Part print with two shaded views. Sizes in mm from the minimum x, y, z corner. Coordinates: 2 decimals unless noted, no trailing zeros. Loops run counter-clockwise (first coordinate to the right, second up) from the corner with the lowest first, then second, coordinate; pieces in that order, holes last. Notation, with made-up numbers: (24, 78.25) -> (57, 78.25) arc R7 cw to (57, 88.25) -> close; hole circle Ø1 at (-34, 76.25). An arc over 180 degrees is marked (long way). Use one line per item in the form item = value.
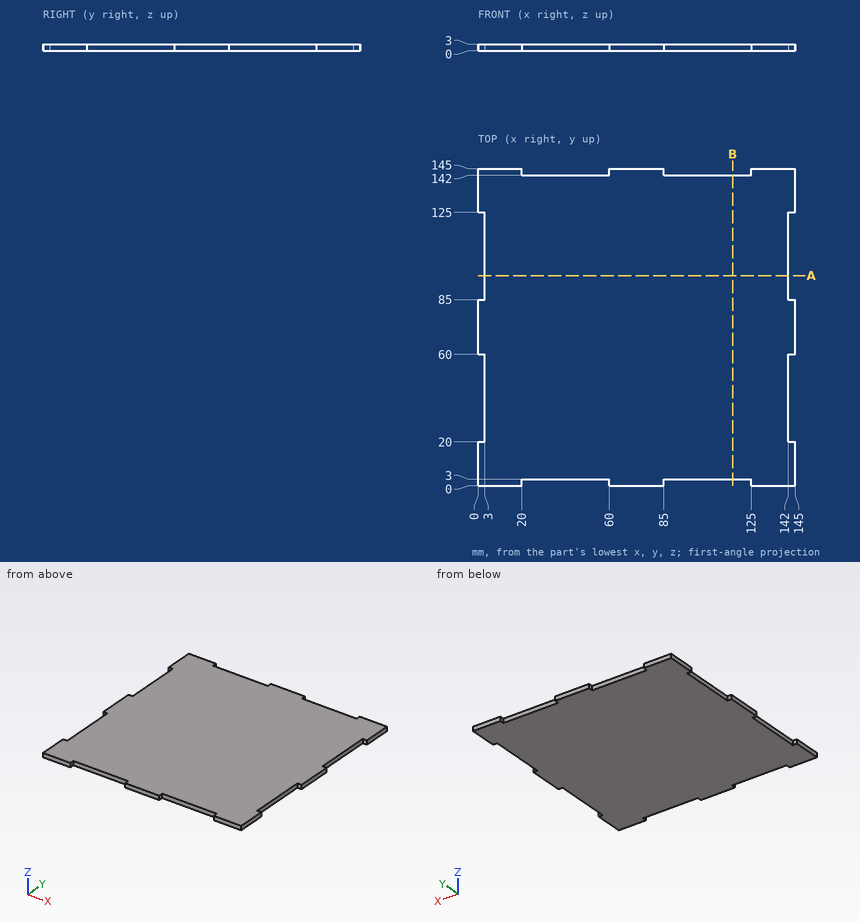
Q1. Band-saw the part on A-A, the plane y = 96. Write the cut outline in (x, z).
Result:
outline = (3, 0) -> (142, 0) -> (142, 3) -> (3, 3) -> close
Q2. Pin check, flat tips, straight feed: pin 1 Ø1 at (x, z) = (28, 2) entering from +Y; pin 2 Ø1.5 at (y, z) = (38.5, 2) entering from -X. Stop position of each tip, or through.
Result:
pin_1 = 142
pin_2 = 3
Q3. Wall check: line 1 along X through (y, z) = (25, 1.6). Give the ranges that are in metal, low to high.
Result:
line_1 = 3 to 142
